Here's how the part is built. I have some questions about the finished solid (model axes, mm). A direction names the side the tool comes from. Round coordinates to 2 decimals unless told otherwise and drop trailing zeros. Loops run counter-clockwise (first coordinate to the right, second up) from the corner with the lowest first, then second, coordinate; pieces in that order, holes last. Notation, with made-up numbers: M 2.25,77 L 29.25,77 A27 ccw 29.25,106 Z; hole C -26,-17 d6. An arc over 180 degrees is marked long. Write each question's results on one line, items separated by ' | '. Start each with the question number.
Autodesk Inventor part; units mm, degrees
ref_plane "YZ Plane" through (0, 0, 0) normal (1, 0, 0) x (0, 1, 0)
ref_plane "XZ Plane" through (0, 0, 0) normal (0, 1, 0) x (-1, 0, 0)
ref_plane "XY Plane" through (0, 0, 0) normal (0, 0, 1) x (1, 0, 0)
sketch "Sketch1" plane through (0, 0, 0) normal (0, 1, 0) x (-1, 0, 0)
  circle A0 centre (0, 0) radius 31.75
  dimension "od" = 63.5
extrude "Extrusion1" add sketch "Sketch1" against normal blind 2.54
sketch "Sketch2" plane through (0, 0, 0) normal (0, 1, 0) x (1, 0, 0)
  line L0 (-7.7063, 0) -> (-3.8531, 6.6738)
  line L1 (-3.8531, 6.6738) -> (3.8531, 6.6738)
  line L2 (3.8531, 6.6738) -> (7.7063, 0)
  line L3 (7.7063, 0) -> (3.8531, -6.6738)
  line L4 (3.8531, -6.6738) -> (-3.8531, -6.6738)
  line L5 (-3.8531, -6.6738) -> (-7.7063, 0)
  point P0 (0, 0)
  point P1 (0, 0)
  dimension "d3" = 13.3477
extrude "Extrusion2" cut sketch "Sketch2" against normal through all
chamfer "Chamfer1" distance 0.7937 angle 45 6 edges at (-5.7797, 0, -3.3369) (0, 0, -6.6738) (5.7797, 0, -3.3369) (5.7797, 0, 3.3369) (0, 0, 6.6738) (-5.7797, 0, 3.3369)
sketch "Sketch4" plane through (0, -2.54, 0) normal (0, -1, 0) x (1, 0, 0)
  circle A0 centre (0, 0) radius 13.589
  circle A1 centre (0, 0) radius 31.75
extrude "Extrusion4" cut sketch "Sketch4" against normal through all
properties part number "spacerForEndV03" material "PC/ABS Plastic"
Item 1: If we section it at C-C on x = 0: Please give me the cut outline in (y, z).
Item 2: If we section it at A-A on y = -1.75: Please give me the cut outline in (x, z).
Item 3: If we mould it in two halves opening along Z, with no side actions, what happens to faces 1 (the face through (6.088, -0.402, 3.585)), 2 (the face through (12.96, -1.29, 4.08)), 3 (the face through (-6, 0, -6))? For each: released by +Z, released by -Z, zero draft, split by the parting line, or undercut.
Item 4: I'm going to push a flat-ended pin straight in: pin 1 (0.5 mm diameter, centred on x = -1, y = -1.5, fed in from +Z). Where does the tip first touch, or does it pass through?
Item 5: Which directions (+Z, -Z, +X, -X, +Y, -Y) give clear straight access to the entire face, cutting with the end or side of a thin tool? Please do faces 4 (the face through (0, -2, 6.674)), 5 (the face through (6.2, -2.54, 3.2)), 6 (the face through (6.15, -0.4, -3.48)).
Item 6: If we section it at B-B on z = 0.75: Please give me the cut outline in (x, y), and give its area (3 significant figures).
Item 7: I need wall thicknesses on L1, parallel to Z at x = -6, y = -1.5; L2, parallel to Z at x = -1.25, y = -1.05; L3, parallel to X at y = -1.65, z = 1.5. Which ranges of each line are inside material? Lowest first, please.
Item 8: If we section it at D-D on z = 10.25: Please give me the cut outline in (x, y).
Numbers:
1) outline: M -2.54,-13.59 L 0,-13.59 L 0,-7.47 L -0.79,-6.67 L -2.54,-6.67 Z; M -2.54,6.67 L -0.79,6.67 L 0,7.47 L 0,13.59 L -2.54,13.59 Z
2) outline: C 0,0 d27.18; hole M -7.71,0 L -3.85,-6.67 L 3.85,-6.67 L 7.71,0 L 3.85,6.67 L -3.85,6.67 Z
3) face 1: undercut | face 2: split by the parting line | face 3: zero draft
4) pin 1: z = 13.57
5) face 4: +Y, -Y | face 5: +Z, -Z, +X, -X, -Y | face 6: +Y
6) outline: M -13.57,-2.54 L -7.27,-2.54 L -7.27,-0.79 L -8.19,0 L -13.57,0 Z; M 7.27,-2.54 L 13.57,-2.54 L 13.57,0 L 8.19,0 L 7.27,-0.79 Z | area: 31.3 mm²
7) L1: -12.19 to -2.96, 2.96 to 12.19 | L2: -13.53 to -6.67, 6.67 to 13.53 | L3: -13.51 to -6.84, 6.84 to 13.51
8) outline: M -8.92,-2.54 L 8.92,-2.54 L 8.92,0 L -8.92,0 Z
